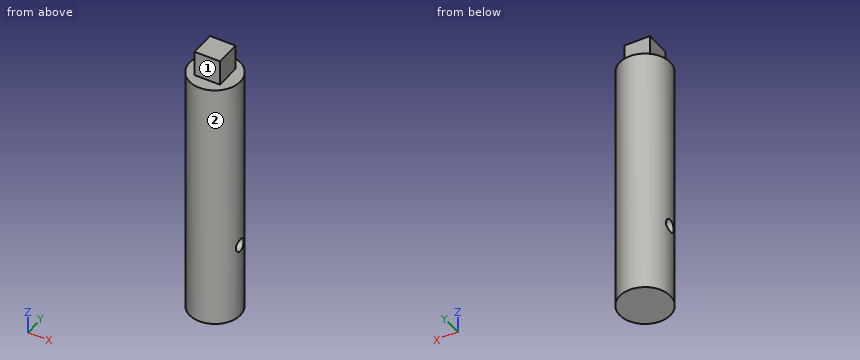
```python
from build123d import *

# Parameters (mm, degrees)
SKETCH1_R               = 5
BOSS_EXTRUDE1_DEPTH     = 50
SKETCH2_W               = 5
SKETCH2_H               = 5
BOSS_EXTRUDE2_DEPTH     = 5
CUT_EXTRUDE1_DEPTH      = 5
CUT_EXTRUDE1_DEPTH_BACK = 5
SKETCH5_R               = 1.25


with BuildPart() as part:
    # Sketch1 → Boss-Extrude1 (new body)
    with BuildSketch(Plane.XY):
        Circle(SKETCH1_R)
    extrude(amount=BOSS_EXTRUDE1_DEPTH)

    # Sketch2 → Boss-Extrude2 (add)
    with BuildSketch(Plane.XY.offset(50)):
        Rectangle(SKETCH2_W, SKETCH2_H)
    extrude(amount=BOSS_EXTRUDE2_DEPTH)

    # Sketch5 → Cut-Extrude1 (cut, two sides: drawn at the far end of the back side and taken through both)
    with BuildSketch(Plane(origin=(0, 0, 0), x_dir=(0, 0, -1), z_dir=(1, 0, 0)).offset(-CUT_EXTRUDE1_DEPTH_BACK)):
        with Locations(Location((-15, 0, 0), (0, 0, 180))):
            Circle(SKETCH5_R)
    extrude(amount=CUT_EXTRUDE1_DEPTH + CUT_EXTRUDE1_DEPTH_BACK, mode=Mode.SUBTRACT)


solid = part.part
```
Build history of the part. All positions in model axes, mm. Face numbers are marked on the shaded views. A direction names the side the tool comes from. Round coordinates to 2 decimals unless told otherwise and drop trailing zeros. Write each loop counter-clockwise with the first axis right and the second up, starting at its lowest first coordinate (ties: lowest second). Pieces come first, ordered by that corner, then holes. Notation, with made-up numbers: (7.25, 29.25) - (21.25, 29.25) arc R31 cw to (21.25, 60.25) - close; hole circle Ø8 at (-1, 89). An arc over 180 degrees is marked (long way). Write each question's results on one line, items separated by ' | '. Start each with the question number.
Item 1: Wall check: L1, parallel to Y at x = -0.25, z = 15; L2, parallel to X at y = -0.25, z = 48.5; L3, parallel to Y at x = -2.25, z = 50.5. Give the ranges that are in metal, low to high. Write a range as [from, to].
Item 2: Saw through at B-B (x = 0). Write the cut outline in (y, z), and give its area (3 significant figures).
Item 3: Saw through at A-A (y = 0). Write the cut outline in (x, z), and give its area (3 significant figures).
Item 4: Which spindle directions (+Z, -Z, +X, -X, +Y, -Y) get a long thin tool onto all of the face, cutting with end or side? Do the marked faces 1 and 2. Say none if no direction does.
Item 5: Saw through at D-D (y = 2). Write the cut outline in (x, z), and give its area (3 significant figures).
Item 6: Drop flat-ended pins along their axis: P1, Ø1.5, axis at x = 3.5, z = 12.5, coming from the +Y side; P2, Ø1.5, axis at y = 0.5, z = 52, coming from the +X side; P3, Ø4, axis at y = 1, z = 52.5, coming from the -X side; P4, Ø2, axis at y = 0, z = 15, coming from the -X side. Give the stop position or say it passes through.
Item 7: Saw through at C-C (z = 19). Write the cut outline in (x, y).
Results are:
1) L1: y = [-4.99, -1.25], [1.25, 4.99] | L2: x = [-4.99, 4.99] | L3: y = [-2.5, 2.5]
2) outline: (-5, 0) - (5, 0) - (5, 50) - (2.5, 50) - (2.5, 55) - (-2.5, 55) - (-2.5, 50) - (-5, 50) - close; hole circle Ø2.5 at (0, 15) | area: 520 mm²
3) outline: (-5, 0) - (5, 0) - (5, 13.75) - (-5, 13.75) - close; (-5, 16.25) - (5, 16.25) - (5, 50) - (2.5, 50) - (2.5, 55) - (-2.5, 55) - (-2.5, 50) - (-5, 50) - close | area: 500 mm²
4) face 1: +Z, +X, -X, -Y | face 2: +Z, -Z
5) outline: (-4.58, 0) - (4.58, 0) - (4.58, 50) - (2.5, 50) - (2.5, 55) - (-2.5, 55) - (-2.5, 50) - (-4.58, 50) - close | area: 483 mm²
6) P1: stops at y = 4.18 | P2: stops at x = 2.5 | P3: stops at x = -2.5 | P4: passes through
7) outline: circle Ø10 at (0, 0)
